from build123d import *

# Parameters (mm, degrees)
SKETCH_1_R          = 49
SKETCH_1_R_2        = 40.5
EXTRUDE_1_DEPTH     = 5.5
SKETCH_1_5_R        = 40.5
SKETCH_1_5_R_2      = 36.5
EXTRUDE_2_DEPTH     = 17.8
EXTRUDE_START       = 17.8
SKETCH_1_6_R        = 40.5
SKETCH_1_6_R_2      = 36.5
EXTRUDE_3_DEPTH     = 5
SKETCH_2_R          = 2.2
CUT_EXTRUDE_1_DEPTH = 50
SKETCH_3_R          = 2.2
CUT_EXTRUDE_2_DEPTH = 50
SKETCH_4_W          = 33.937530488
SKETCH_4_H          = 35
CUT_EXTRUDE_3_DEPTH = 11
SKETCH_7_R          = 3.75
CUT_EXTRUDE_5_DEPTH = 1
CHAMFER_8_SIZE      = 0.3
CHAMFER_9_SIZE      = 2
CHAMFER_11_SIZE     = 0.3
SKETCH_8_R          = 3
EXTRUDE_4_DEPTH     = 4
CHAMFER_START       = 17.800013545
CHAMFER_12_2_DEPTH  = 4.999986455
CUT_EXTRUDE_8_DEPTH = 10
CHAMFER_13_SIZE     = 0.3
SKETCH_2_3_R        = 2
CUT_EXTRUDE_9_DEPTH = 4.5
CHAMFER_10_SIZE     = 0.3


with BuildPart() as part:
    # 스케치1 → 보스-돌출1 (new body)
    with BuildSketch(Plane(origin=(0, 0, 0), x_dir=(1, 0, 0), z_dir=(0, 1, 0))):
        with Locations(Location((0, 0, 0), (0, 0, 270))):
            Circle(SKETCH_1_R)
        with Locations(Location((0, 0, 0), (0, 0, 270))):
            Circle(SKETCH_1_R_2, mode=Mode.SUBTRACT)
    extrude(amount=EXTRUDE_1_DEPTH)

    # 스케치1<5> → 보스-돌출2 (add)
    with BuildSketch(Plane(origin=(0, 0, 0), x_dir=(1, 0, 0), z_dir=(0, 1, 0))):
        with Locations(Location((0, 0, 0), (0, 0, 270))):
            Circle(SKETCH_1_5_R)
        with Locations(Location((0, 0, 0), (0, 0, 270))):
            Circle(SKETCH_1_5_R_2, mode=Mode.SUBTRACT)
    extrude(amount=EXTRUDE_2_DEPTH)

    # 스케치1<6> → 보스-돌출3 (add)
    # profile 1 of 2: a face of its own
    with BuildSketch(Plane(origin=(0, 0, 0), x_dir=(1, 0, 0), z_dir=(0, 1, 0)).offset(EXTRUDE_START)):
        with Locations(Location((0, 0, 0), (0, 0, 270))):
            Circle(SKETCH_1_6_R)
        with Locations(Location((0, 0, 0), (0, 0, 270))):
            Circle(SKETCH_1_6_R_2, mode=Mode.SUBTRACT)
    # profile 2 of 2: a face of its own
    with BuildSketch(Plane(origin=(0, 0, 0), x_dir=(1, 0, 0), z_dir=(0, 1, 0)).offset(EXTRUDE_START)):
        with Locations(Location((0, 0, 0), (0, 0, 270))):
            Circle(SKETCH_1_6_R_2)
    extrude(amount=EXTRUDE_3_DEPTH)

    # 스케치2 → 컷-돌출1 (cut)
    with BuildSketch(Plane(origin=(0, 22.8, 0), x_dir=(1, 0, 0), z_dir=(0, 1, 0))):
        with Locations(Location((0, 12, 0), (0, 0, 270))):
            Circle(SKETCH_2_R)
        with Locations(Location((10.392304845, 6, 0), (0, 0, 270))):
            Circle(SKETCH_2_R)
        with Locations(Location((10.392304845, -6, 0), (0, 0, 270))):
            Circle(SKETCH_2_R)
        with Locations(Location((0, -12, 0), (0, 0, 270))):
            Circle(SKETCH_2_R)
        with Locations(Location((-10.392304845, -6, 0), (0, 0, 270))):
            Circle(SKETCH_2_R)
        with Locations(Location((-10.392304845, 6, 0), (0, 0, 270))):
            Circle(SKETCH_2_R)
    extrude(amount=-CUT_EXTRUDE_1_DEPTH, mode=Mode.SUBTRACT)

    # 스케치3 → 컷-돌출2 (cut)
    with BuildSketch(Plane(origin=(0, 5.5, 0), x_dir=(1, 0, 0), z_dir=(0, 1, 0))):
        with Locations(Location((-43.846652915, 10.122797445, 0), (0, 0, 270))):
            Circle(SKETCH_3_R)
        with Locations(Location((-13.156726713, 43.033714018, 0), (0, 0, 270))):
            Circle(SKETCH_3_R)
        with Locations(Location((30.689926203, 32.910916573, 0), (0, 0, 270))):
            Circle(SKETCH_3_R)
        with Locations(Location((43.846652915, -10.122797445, 0), (0, 0, 270))):
            Circle(SKETCH_3_R)
        with Locations(Location((13.156726713, -43.033714018, 0), (0, 0, 270))):
            Circle(SKETCH_3_R)
        with Locations(Location((-30.689926203, -32.910916573, 0), (0, 0, 270))):
            Circle(SKETCH_3_R)
    extrude(amount=-CUT_EXTRUDE_2_DEPTH, mode=Mode.SUBTRACT)

    # 스케치4 → 컷-돌출3 (cut)
    with BuildSketch(Plane.XZ):
        with Locations((-49, 0)):
            Rectangle(SKETCH_4_W, SKETCH_4_H)
    extrude(amount=-CUT_EXTRUDE_3_DEPTH, mode=Mode.SUBTRACT)

    # 스케치7 → 컷-돌출5 (cut)
    with BuildSketch(Plane(origin=(0, 5.5, 0), x_dir=(1, 0, 0), z_dir=(0, 1, 0))):
        with Locations(Location((-13.156726713, 43.033714018, 0), (0, 0, 270))):
            Circle(SKETCH_7_R)
        with Locations(Location((30.689926203, 32.910916573, 0), (0, 0, 270))):
            Circle(SKETCH_7_R)
        with Locations(Location((43.846652915, -10.122797445, 0), (0, 0, 270))):
            Circle(SKETCH_7_R)
        with Locations(Location((13.156726713, -43.033714018, 0), (0, 0, 270))):
            Circle(SKETCH_7_R)
        with Locations(Location((-30.689926203, -32.910916573, 0), (0, 0, 270))):
            Circle(SKETCH_7_R)
        with Locations((-43.846652915, 10.122797445)):
            Circle(SKETCH_7_R)
    extrude(amount=-CUT_EXTRUDE_5_DEPTH, mode=Mode.SUBTRACT)

    # 모따기8
    chamfer_8_edges = [part.edges().sort_by_distance(p)[0] for p in [
        (-38.899836832, 0, 17.5),
        (-38.899836832, 0, -17.5),
        (0, 17.8, -36.5),
        (31.392674305, 0, -18.62122445),
        (49, 0, 0),
        (-34.277599746, 11, -17.5),
        (-34.277599746, 11, 17.5),
    ]]
    chamfer(chamfer_8_edges, length=CHAMFER_8_SIZE)

    # 모따기9
    # the kernel refuses this chamfer: 2 mm, written as the material it takes off along each edge
    with BuildSketch(Plane(origin=(0, 5.5, 0), x_dir=(-0.9664639916292301, 0, -0.25680216682126217), z_dir=(-0.25680216682126217, 0, 0.9664639916292301))) as chamfer_9_piece_1:
        Polygon((49, CHAMFER_9_SIZE), (49 - CHAMFER_9_SIZE, 0), (49, 0), align=None)
    revolve(axis=Axis((0, 5.5, 0), (0, -1, 0)), revolution_arc=330.239203437, mode=Mode.SUBTRACT)

    # 모따기11
    chamfer_11_edges = [part.edges().sort_by_distance(p)[0] for p in [
        (34.270978976, 5.5, -21.581241855),
    ]]
    chamfer(chamfer_11_edges, length=CHAMFER_11_SIZE)

    # 스케치8 → 보스-돌출4 (add)
    with BuildSketch(Plane(origin=(0, 22.8, 0), x_dir=(1, 0, 0), z_dir=(0, 1, 0))):
        with Locations((10.963938927, -35.861428349)):
            Circle(SKETCH_8_R)
        with BuildLine():
            Line((11.493879557, -27.333875187), (5.756051021, -29.088105415))
            Line((5.756051021, -29.088105415), (8.095024659, -36.738543463))
            ThreePointArc((8.095024659, -36.738543463), (10.086823813, -32.992514081), (13.832853195, -34.984313234))
            Line((13.832853195, -34.984313234), (11.493879557, -27.333875187))
        make_face()
    extrude(amount=EXTRUDE_4_DEPTH)

    # 모따기12: read off the stored shape, not the designer's step
    # 모따기12 outline → 모따기12 (revolve, cut)
    with BuildSketch(Plane.XY):
        Polygon((40.5, 22.8), (35.5, 22.8), (40.5, 17.8), align=None)
    revolve(axis=Axis((0, 0, 0), (0, 1, 0)), mode=Mode.SUBTRACT)

    # Chamfer 12 2 outline → Chamfer 12 2 (add)
    with BuildSketch(Plane(origin=(0, 0, 0), x_dir=(1, 0, 0), z_dir=(0, 1, 0)).offset(CHAMFER_START)):
        with BuildLine():
            ThreePointArc((8.095024659, -36.738543463), (11.841054042, -38.730342617), (13.832853195, -34.984313234))
            Line((13.832853195, -34.984313234), (12.614726395, -31))
            Line((12.614726395, -31), (6.340575855, -31))
            Line((6.340575855, -31), (8.095024659, -36.738543463))
        make_face()
    extrude(amount=CHAMFER_12_2_DEPTH)

    # 스케치10 → 컷-돌출8 (cut)
    with BuildSketch(Plane(origin=(-2.868914268, 0, 0.877115114), x_dir=(0.29237170472273827, 0, 0.9563047559630351), z_dir=(-0.9563047559630351, 0, 0.29237170472273827))):
        Polygon((29.5, 22.8), (33.5, 26.8), (29.5, 26.8), align=None)
    extrude(amount=-CUT_EXTRUDE_8_DEPTH, mode=Mode.SUBTRACT)

    # 모따기13
    chamfer_13_edges = [part.edges().sort_by_distance(p)[0] for p in [
        (11.841054041, 26.8, 38.730342617),
        (13.248109786, 26.8, 33.071703723),
        (7.51028125, 26.8, 34.825933951),
        (12.078622967, 24.8, 29.246484699),
        (6.340794431, 24.8, 31.000714927),
    ]]
    chamfer(chamfer_13_edges, length=CHAMFER_13_SIZE)

    # 스케치2<3> → 컷-돌출9 (cut)
    with BuildSketch(Plane(origin=(0, 22.8, 0), x_dir=(1, 0, 0), z_dir=(0, 1, 0))):
        with Locations(Location((6, 10.392304845, 0), (0, 0, 270))):
            Circle(SKETCH_2_3_R)
        with Locations(Location((-6, -10.392304845, 0), (0, 0, 270))):
            Circle(SKETCH_2_3_R)
    extrude(amount=-CUT_EXTRUDE_9_DEPTH, mode=Mode.SUBTRACT)

    # 모따기10
    chamfer_10_edges = [part.edges().sort_by_distance(p)[0] for p in [
        (28.132432353, 5.5, -30.168340192),
        (40.192765172, 5.5, 9.279230992),
        (12.06033282, 5.5, 39.447571183),
        (-28.132432353, 5.5, 30.168340192),
        (-12.06033282, 5.5, -39.447571183),
        (0, 17.8, -14.2),
        (-10.392304845, 17.8, -8.2),
        (-10.392304845, 17.8, 3.8),
        (0, 17.8, 9.8),
        (10.392304845, 17.8, -8.2),
        (10.392304845, 17.8, 3.8),
        (0, 22.8, -14.2),
        (-10.392304845, 22.8, -8.2),
        (-10.392304845, 22.8, 3.8),
        (-6, 22.8, 8.392304845),
        (0, 22.8, 9.8),
        (10.392304845, 22.8, 3.8),
        (6, 22.8, -12.392304845),
        (10.392304845, 22.8, -8.2),
    ]]
    chamfer(chamfer_10_edges, length=CHAMFER_10_SIZE)


solid = part.part
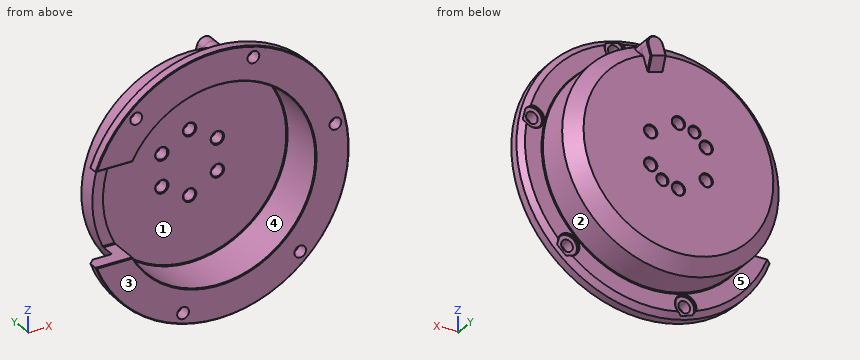
For this review, take the finished solid that the model builds, in its own axes (mm). Face numbers are marked on the shaded views. A direction names the side the tool comes from. Round coordinates to 2 decimals unless told otherwise and drop trailing zeros. One line per question, with ' | ' between items.
Q1. The part is to be moulded in two halves that separate along Z. For the marked faces 1, 2 and 3, say which applies: released by +Z, released by -Z, zero draft, split by the parting line, or undercut.
Taken from the geometry:
face 1: undercut | face 2: split by the parting line | face 3: zero draft
Q2. For pin 1 (4 mm diameter, centred on x = 31, z = -31.5, fed in from +Y); pin 2 (12 mm diameter, centred on y = 19, z = 21.5, fed in from +X); pin 3 (3.5 mm diameter, centred on x = 30.69, z = -32.91, fed in from +Y); pin 4 (10 mm diameter, centred on x = 25, y = 15, fed in from +Z), all flat-tipped, find the tip position at first contact; note any pin that passes through.
Taken from the geometry:
pin 1: stops at y = 4.5 | pin 2: stops at x = 37.37 | pin 3: passes through | pin 4: stops at z = 35.22
Q3. Take a section at A-A (x = 0). State how many separate pieces and enclosed holes the cut face has, and give its area (3 significant figures).
Taken from the geometry:
separate pieces: 3 | enclosed holes: 0 | area: 568 mm²
Q4. For line 1 along Y through (x, z) = (-4, -16); line 2 along Y through (x, z) = (-36, 24.5); line 3 along X through (y, z) = (17.75, 18), list the stretches that pass through material, from the lowest coordinate up. Write a range as [from, to].
Taken from the geometry:
line 1: y = [17.8, 22.8] | line 2: y = [0, 5.5] | line 3: x = [-36.28, -31.47], [31.47, 36.28]
Q5. Tool access review of the marked faces 4 and 5: name each direction out of +Z, -Z, +X, -X, +Y, -Y from which nothing blocks a thin tool from reaching the whole face with its end or side.
Taken from the geometry:
face 4: -Y | face 5: +Y
